```python
from build123d import *

# Parameters (mm, degrees)
SKETCH1_W                                        = 114.3
SKETCH1_H                                        = 114.3
BOSS_EXTRUDE1_DEPTH                              = 12.7
CBORE_FOR_1_4_SOCKET_HEAD_CAP_SCREW1_D           = 6.5278
CBORE_FOR_1_4_SOCKET_HEAD_CAP_SCREW1_CBORE_D     = 11.1125
CBORE_FOR_1_4_SOCKET_HEAD_CAP_SCREW1_CBORE_DEPTH = 6.35
T_SLOT_CUT_WITH_MCMASTER_8789A16_BIT_DEPTH       = 129.420802443
FILLET1_R                                        = 6.35


with BuildPart() as part:
    # Sketch1 → Boss-Extrude1 (new body)
    with BuildSketch(Plane(origin=(0, 0, 0), x_dir=(1, 0, 0), z_dir=(0, 1, 0))):
        Rectangle(SKETCH1_W, SKETCH1_H)
    extrude(amount=BOSS_EXTRUDE1_DEPTH)

    # CBORE for 1/4 Socket Head Cap Screw1 (through all)
    with Locations(Plane(origin=(0, 12.7, 0), x_dir=(1, 0, 0), z_dir=(0, 1, 0))):
        with Locations((-47.625, 47.625), (47.625, 47.625), (47.625, -47.625), (-47.625, -47.625)):
            CounterBoreHole(CBORE_FOR_1_4_SOCKET_HEAD_CAP_SCREW1_D / 2, CBORE_FOR_1_4_SOCKET_HEAD_CAP_SCREW1_CBORE_D / 2, CBORE_FOR_1_4_SOCKET_HEAD_CAP_SCREW1_CBORE_DEPTH)

    # Sketch4 → T-SLOT CUT WITH MCMASTER 8789A16 BIT (cut, through all)
    with BuildSketch(Plane.XY.offset(57.15)):
        Polygon((-31.9484375, 12.7), (-31.9484375, 9.525), (-35.71875, 9.525), (-35.71875, 3.571875), (-21.43125, 3.571875), (-21.43125, 9.525), (-25.2015625, 9.525), (-25.2015625, 12.7), align=None)
        Polygon((25.2015625, 9.525), (25.2015625, 12.7), (31.9484375, 12.7), (31.9484375, 9.525), (35.71875, 9.525), (35.71875, 3.571875), (21.43125, 3.571875), (21.43125, 9.525), align=None)
    extrude(amount=-T_SLOT_CUT_WITH_MCMASTER_8789A16_BIT_DEPTH, mode=Mode.SUBTRACT)

    # Fillet1
    fillet1_edges = [part.edges().sort_by_distance(p)[0] for p in [
        (57.15, 6.35, 57.15),
        (-57.15, 6.35, 57.15),
        (-57.15, 6.35, -57.15),
        (57.15, 6.35, -57.15),
    ]]
    fillet(fillet1_edges, radius=FILLET1_R)


solid = part.part
```
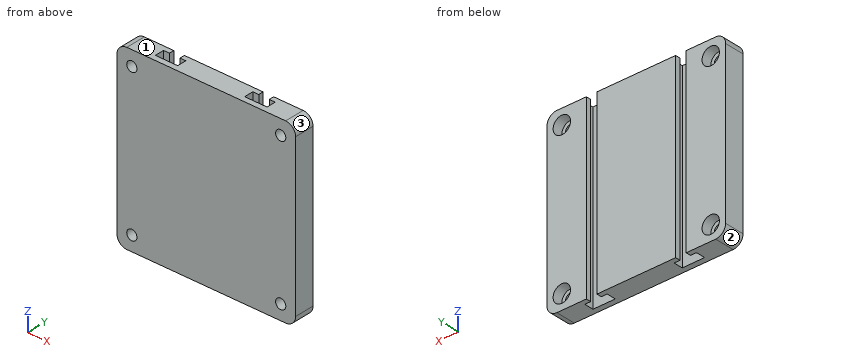
The listing builds one solid part. Answer for the finished solid, in the listing's coordinates (mm). Face numbers are marked on the shaded views. Coordinates: 2 decimals unless noted, no trailing zeros. Loops run counter-clockwise (first coordinate to the right, second up) from the corner with the lowest first, then second, coordinate; pieces in that order, holes last. Notation, with made-up numbers: (24, 74) - (57, 74) arc R17 ccw to (57, 89) - close; hole circle Ø6 at (9.25, 3). An arc over 180 degrees is marked (long way). Use a Markdown table: item, result. Add a question column.
1) The part is cut by section C-C, the plane z = 17. Give the vertices of the cut face in (x, y) (3 decimals), and give its area (3 significant figures).
2) The part is cut by section A-A, the plane x = -23. Give the vertices of the cut face in (y, z) (3 decimals), and give its area (3 significant figures).
3) The mould has two halves that part along X. Classify the marked faces 1, 2 and 3: released by +X, released by -X, zero draft, split by the parting line, or undercut.
4) The part is cut by section B-B, the plane x = -49. Give the vertices of the cut face in (y, z), and give its area (3 significant figures).
5) Find the intervals of material crossed by line 1 (X direction, y = 6, z = 43.5); line 2 (X direction, y = 10.5, z = -27); line 3 (Y direction, x = -24, z = 47) (3 decimals), in increasing order.
6) Given pin 1 (5.5 mm diameter, centred on x = 45.5, z = -46.5, fed in from +Y); pin 2 (1.5 mm diameter, centred on x = 23, y = 5, fed in from +Z), each flat-ended and moving along its own axis, determine where each tip first touches the part or whether it passes through.
Here are the results:
| question | item | result |
|---|---|---|
| 1 | outline | (-57.15, 0) - (57.15, 0) - (57.15, 12.7) - (31.948, 12.7) - (31.948, 9.525) - (35.719, 9.525) - (35.719, 3.572) - (21.431, 3.572) - (21.431, 9.525) - (25.202, 9.525) - (25.202, 12.7) - (-25.202, 12.7) - (-25.202, 9.525) - (-21.431, 9.525) - (-21.431, 3.572) - (-35.719, 3.572) - (-35.719, 9.525) - (-31.948, 9.525) - (-31.948, 12.7) - (-57.15, 12.7) - close |
| 1 | area | 1,240 mm^2 |
| 2 | outline | (0, -57.15) - (3.572, -57.15) - (3.572, 57.15) - (0, 57.15) - close; (9.525, -57.15) - (12.7, -57.15) - (12.7, 57.15) - (9.525, 57.15) - close |
| 2 | area | 771 mm^2 |
| 3 | face 1 | zero draft |
| 3 | face 2 | released by -X |
| 3 | face 3 | released by +X |
| 4 | outline | (0, -57.15) - (12.7, -57.15) - (12.7, -53.01) - (6.35, -53.01) - (6.35, -50.59) - (0, -50.59) - close; (0, -44.66) - (6.35, -44.66) - (6.35, -42.24) - (12.7, -42.24) - (12.7, 42.24) - (6.35, 42.24) - (6.35, 44.66) - (0, 44.66) - close; (0, 50.59) - (6.35, 50.59) - (6.35, 53.01) - (12.7, 53.01) - (12.7, 57.15) - (0, 57.15) - close |
| 4 | area | 1,240 mm^2 |
| 5 | line 1 | x = -57.15 to -35.72, -21.43 to 21.43, 35.72 to 57.15 |
| 5 | line 2 | x = -57.15 to -31.95, -25.2 to 25.2, 31.95 to 57.15 |
| 5 | line 3 | y = 0 to 3.572, 9.525 to 12.7 |
| 6 | pin 1 | stops at y = 6.35 |
| 6 | pin 2 | passes through |
